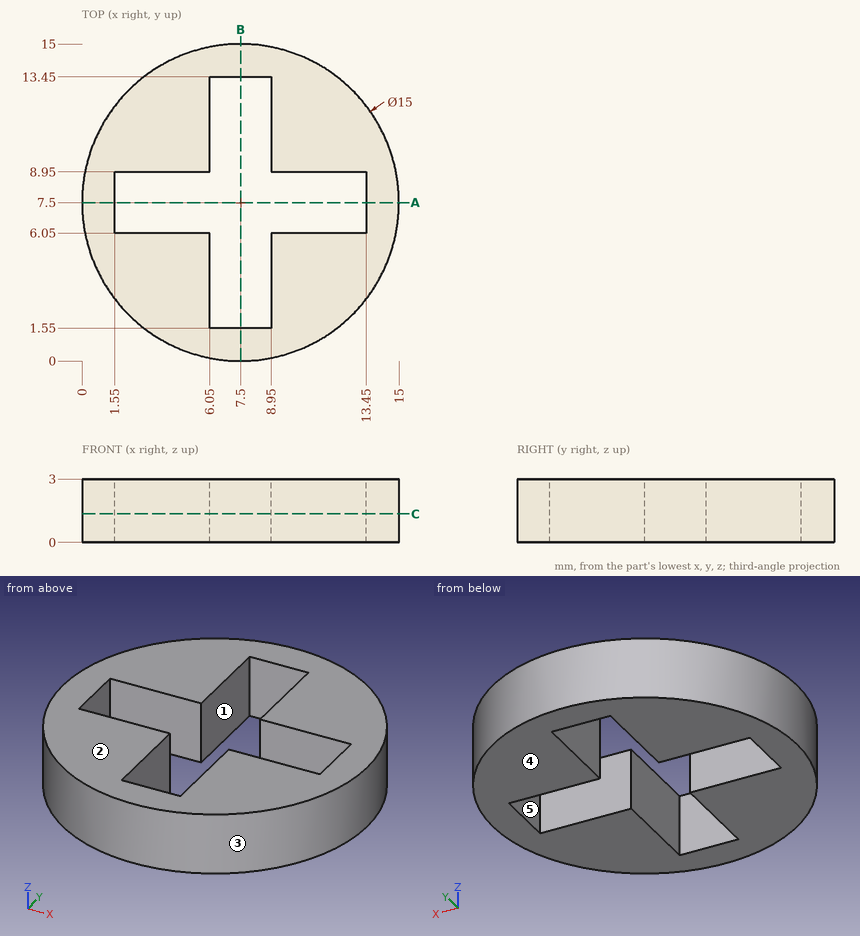
Geometry check sheet. Reference: drawing and pictorial views, mm from the part's lowest x, y, z. A direction names the side the tool comes from. Round coordinates to 2 decimals unless told otherwise and drop trailing zeros. Order: outer loops, then holes, each group sorted by start corner. A loop starts at its lowest first (then second) coordinate and runs counter-clockwise, first axis right, second up. Notation, with made-up numbers: (56.25, 30) - (67.25, 30) arc R18 cw to (67.25, 45) - close; hole circle Ø1 at (72.25, -24.75). An arc over 180 degrees is marked (long way). Write item = value, one per line.
Q1. Tool access check on the marked faces 4 and 5. Record the directions out of +Z, -Z, +X, -X, +Y, -Y that give a thin tool (end or side, any length) a straight path to the whole face; none if there is none.
Computed:
face_4 = -Z, +X, -X, +Y, -Y
face_5 = +Z, -Z
Q2. Section check A-A (y = 7.5). Record the boundary of the cut face in (x, z), and give its area (3 significant figures).
Computed:
outline = (0, 0) - (1.55, 0) - (1.55, 3) - (0, 3) - close; (13.45, 0) - (15, 0) - (15, 3) - (13.45, 3) - close
area = 9.30 mm^2
Q3. Thickness scan on line 1 along Y through (x, z) = (13, 1.55); line 2 along X through (y, z) = (6, 1.85); line 3 along X through (y, z) = (6.5, 1.65). Record the ranges inside material, lowest first.
Computed:
line_1 = 2.4 to 6.05, 8.95 to 12.6
line_2 = 0.15 to 6.05, 8.95 to 14.85
line_3 = 0.07 to 1.55, 13.45 to 14.93
Q4. Section check C-C (z = 1.35). Record the boundary of the cut face in (x, y).
Computed:
outline = circle Ø15 at (7.5, 7.5); hole (1.55, 6.05) - (6.05, 6.05) - (6.05, 1.55) - (8.95, 1.55) - (8.95, 6.05) - (13.45, 6.05) - (13.45, 8.95) - (8.95, 8.95) - (8.95, 13.45) - (6.05, 13.45) - (6.05, 8.95) - (1.55, 8.95) - close
Q5. Go/stop test with a flat-tipped pin: pin 1 (1 mm diameter, centred on y = 8.5, z = 1, fed in from -X). Record where the tip stops, or that it passes through.
Computed:
pin_1 = 0.02
Q6. Draft check along X on the marked faces 1, 2 and 3. Enter one of: pulls with the +X half, pulls with the -X half, needs draft (parallel to the pull), parting line crosses it, or undercut.
Computed:
face_1 = undercut
face_2 = needs draft
face_3 = parting line crosses it
